For this review, take the finished solid that the model builds, in its own axes (mm). Face numbers are marked on the shaded views. A direction names the side the tool comes from. Give positions to 0.01 mm unless a question says otherwise; leave off trailing zeros. Loops run counter-clockwise (first coordinate to the right, second up) from the corner with the lowest first, then second, coordinate; pieces in that order, holes last. Notation, with made-up numbers: (29, -21.5) - (63, -21.5) arc R22 cw to (63, -10.5) - close; hole circle Ø4 at (83.25, -19). An arc over 180 degrees is marked (long way). Put each result on its own line as item: value.
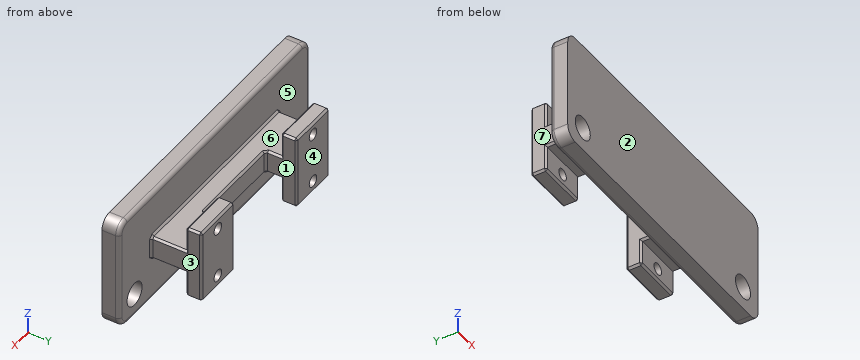
from build123d import *

# Parameters (mm, degrees)
SKETCH1_R                = 3
BOSS_EXTRUDE1_DEPTH      = 4.5
BOSS_EXTRUDE2_DEPTH      = 25.5
BOSS_EXTRUDE2_DEPTH_BACK = 25.5
CUT_EXTRUDE1_DEPTH       = 9.5
CUT_EXTRUDE1_DEPTH_BACK  = 9.5
SKETCH3_W                = 25
SKETCH3_H                = 16
CUT_EXTRUDE2_REACH       = 46.278
SKETCH4_R                = 1.5
FILLET1_R                = 1
CHAMFER1_SIZE            = 0.5


with BuildPart() as part:
    # Sketch1 → Boss-Extrude1 (new body)
    with BuildSketch(Plane(origin=(0, 0, 0), x_dir=(1, 0, 0), z_dir=(0, 1, 0))):
        with BuildLine():
            Line((-35, -14.5), (35, -14.5))
            ThreePointArc((35, -14.5), (37.121320344, -13.621320344), (38, -11.5))
            Line((38, -11.5), (38, 11.5))
            ThreePointArc((38, 11.5), (37.121320344, 13.621320344), (35, 14.5))
            Line((35, 14.5), (-35, 14.5))
            ThreePointArc((-35, 14.5), (-37.121320344, 13.621320344), (-38, 11.5))
            Line((-38, 11.5), (-38, -11.5))
            ThreePointArc((-38, -11.5), (-37.121320344, -13.621320344), (-35, -14.5))
        make_face()
        with Locations(Location((-32, 8.5, 0), (0, 0, 270))):
            Circle(SKETCH1_R, mode=Mode.SUBTRACT)
        with Locations(Location((32, 8.5, 0), (0, 0, 270))):
            Circle(SKETCH1_R, mode=Mode.SUBTRACT)
    extrude(amount=BOSS_EXTRUDE1_DEPTH)

    # Sketch2 → Boss-Extrude2 (add, two sides: drawn at the far end of the back side and taken through both)
    with BuildSketch(Plane(origin=(0, 0, 0), x_dir=(0, 0, -1), z_dir=(1, 0, 0)).offset(-BOSS_EXTRUDE2_DEPTH_BACK)):
        Polygon((-3, 4.5), (-3, 13.5), (-9.5, 13.5), (-9.5, 17.5), (9.5, 17.5), (9.5, 13.5), (3, 13.5), (3, 4.5), align=None)
    extrude(amount=BOSS_EXTRUDE2_DEPTH + BOSS_EXTRUDE2_DEPTH_BACK)

    # Sketch3 → Cut-Extrude1 (cut, two sides: drawn at the far end of the back side and taken through both)
    with BuildSketch(Plane.XY.offset(-CUT_EXTRUDE1_DEPTH_BACK)):
        with Locations((0, 17.5)):
            Rectangle(SKETCH3_W, SKETCH3_H)
    extrude(amount=CUT_EXTRUDE1_DEPTH + CUT_EXTRUDE1_DEPTH_BACK, mode=Mode.SUBTRACT)

    # Sketch4 → Cut-Extrude2 (cut, up to next)
    with BuildSketch(Plane(origin=(0, 17.5, 0), x_dir=(1, 0, 0), z_dir=(0, 1, 0)), mode=Mode.PRIVATE) as cut_extrude2_sk1:
        with Locations(Location((-19, 6.5, 0), (0, 0, 270))):
            Circle(SKETCH4_R)
    cut_extrude2_tool1 = extrude(cut_extrude2_sk1.sketch, amount=-CUT_EXTRUDE2_REACH, mode=Mode.PRIVATE) & part.part
    # Sketch4 → Cut-Extrude2 (cut, up to next)
    with BuildSketch(Plane(origin=(0, 17.5, 0), x_dir=(1, 0, 0), z_dir=(0, 1, 0)), mode=Mode.PRIVATE) as cut_extrude2_sk2:
        with Locations(Location((-19, -6.5, 0), (0, 0, 270))):
            Circle(SKETCH4_R)
    cut_extrude2_tool2 = extrude(cut_extrude2_sk2.sketch, amount=-CUT_EXTRUDE2_REACH, mode=Mode.PRIVATE) & part.part
    # Sketch4 → Cut-Extrude2 (cut, up to next)
    with BuildSketch(Plane(origin=(0, 17.5, 0), x_dir=(1, 0, 0), z_dir=(0, 1, 0)), mode=Mode.PRIVATE) as cut_extrude2_sk3:
        with Locations(Location((19, -6.5, 0), (0, 0, 270))):
            Circle(SKETCH4_R)
    cut_extrude2_tool3 = extrude(cut_extrude2_sk3.sketch, amount=-CUT_EXTRUDE2_REACH, mode=Mode.PRIVATE) & part.part
    # Sketch4 → Cut-Extrude2 (cut, up to next)
    with BuildSketch(Plane(origin=(0, 17.5, 0), x_dir=(1, 0, 0), z_dir=(0, 1, 0)), mode=Mode.PRIVATE) as cut_extrude2_sk4:
        with Locations(Location((19, 6.5, 0), (0, 0, 270))):
            Circle(SKETCH4_R)
    cut_extrude2_tool4 = extrude(cut_extrude2_sk4.sketch, amount=-CUT_EXTRUDE2_REACH, mode=Mode.PRIVATE) & part.part
    add(cut_extrude2_tool1.solids().sort_by_distance((-19, 17.5, -6.5))[0], mode=Mode.SUBTRACT)
    add(cut_extrude2_tool2.solids().sort_by_distance((-19, 17.5, 6.5))[0], mode=Mode.SUBTRACT)
    add(cut_extrude2_tool3.solids().sort_by_distance((19, 17.5, 6.5))[0], mode=Mode.SUBTRACT)
    add(cut_extrude2_tool4.solids().sort_by_distance((19, 17.5, -6.5))[0], mode=Mode.SUBTRACT)

    # Fillet1
    fillet1_edges = [part.edges().sort_by_distance(p)[0] for p in [
        (37.121320344, 4.5, 13.621320344),
        (38, 4.5, 0),
        (37.121320344, 4.5, -13.621320344),
        (0, 4.5, -14.5),
        (-37.121320344, 4.5, -13.621320344),
        (-38, 4.5, 0),
        (-37.121320344, 4.5, 13.621320344),
        (0, 4.5, 14.5),
    ]]
    fillet(fillet1_edges, radius=FILLET1_R)

    # Chamfer1
    chamfer1_edges = [part.edges().sort_by_distance(p)[0] for p in [
        (25.5, 9, 3),
        (25.5, 13.5, 6.25),
        (19, 13.5, 9.5),
        (25.5, 15.5, 9.5),
        (19, 17.5, 9.5),
        (25.5, 17.5, 0),
        (19, 17.5, -9.5),
        (25.5, 15.5, -9.5),
        (19, 13.5, -9.5),
        (25.5, 13.5, -6.25),
        (25.5, 9, -3),
        (0, 4.5, -3),
        (25.5, 4.5, 0),
        (0, 4.5, 3),
        (-25.5, 4.5, 0),
        (-25.5, 9, 3),
        (-25.5, 13.5, 6.25),
        (-25.5, 15.5, 9.5),
        (-25.5, 17.5, 0),
        (-25.5, 15.5, -9.5),
        (-25.5, 13.5, -6.25),
        (-25.5, 9, -3),
        (-12.5, 11.5, -3),
        (0, 9.5, -3),
        (12.5, 11.5, -3),
        (-19, 13.5, -9.5),
        (-19, 17.5, -9.5),
        (-19, 17.5, 9.5),
        (-19, 13.5, 9.5),
        (-12.5, 15.5, 9.5),
        (12.5, 15.5, 9.5),
        (12.5, 13.5, 6.25),
        (12.5, 11.5, 3),
        (12.5, 13.5, -6.25),
        (12.5, 15.5, -9.5),
        (12.5, 17.5, 0),
        (12.5, 9.5, 0),
        (0, 9.5, 3),
        (-12.5, 9.5, 0),
        (-12.5, 11.5, 3),
        (-12.5, 13.5, 6.25),
        (-12.5, 17.5, 0),
        (-12.5, 15.5, -9.5),
        (-12.5, 13.5, -6.25),
    ]]
    chamfer(chamfer1_edges, length=CHAMFER1_SIZE)


solid = part.part
1) Take a section at D-D on x = 32. State the section outline as (y, z) points, and give its area (3 significant figures).
Geometry check:
outline: (0, -14.5) - (3.5, -14.5) arc R1 ccw to (4.5, -13.5) - (4.5, -11.5) - (0, -11.5) - close; (0, -5.5) - (4.5, -5.5) - (4.5, 13.5) arc R1 ccw to (3.5, 14.5) - (0, 14.5) - close
area: 103 mm²
2) Take a section at B-B on z = 6.5. State how many separate pieces and enclosed holes the cut face has, and give its area (3 significant figures).
Geometry check:
separate pieces: 5
enclosed holes: 0
area: 421 mm²
3) Draft analysis for pull direction Y (two halves, no side actions). For the marked faces 4, 5, 6 and 7, state which applies: pulls with the +Y half, pulls with the -Y half, needs draft (parallel to the pull), parting line crosses it, or undercut.
Geometry check:
face 4: pulls with the +Y half
face 5: undercut
face 6: undercut
face 7: needs draft
4) Wall thickness on line 1 (X direction, y = 14.5, z = -6.5); line 2 (X direction, y = 1.8, z = -8.5); line 3 (Y direction, x = 11.5, z = -7.75): over which ranges is each line inside the solid? List them lowest first.
Geometry check:
line 1: x = -25.5 to -20.5, -17.5 to -12.5, 12.5 to 17.5, 20.5 to 25.5
line 2: x = -38 to -35, -29 to 29, 35 to 38
line 3: y = 0 to 4.5
5) For the marked faces 1, 2 and 3, list the 3-axis set-ups (+Z, -Z, +X, -X, +Y, -Y) from which the entire face can be reached by the end or side of a thin tool; tool diameter is ignored.
Geometry check:
face 1: +Z, -Z, +Y
face 2: +Z, -Z, +X, -X, -Y
face 3: +Z, -Z, +X, +Y
6) Take a section at C-C on y = 11. State the section outline as (x, z) points.
Geometry check:
outline: (-25.5, -2.5) - (-25, -3) - (-13, -3) - (-12.5, -2.5) - (-12.5, 2.5) - (-13, 3) - (-25, 3) - (-25.5, 2.5) - close; (12.5, -2.5) - (13, -3) - (25, -3) - (25.5, -2.5) - (25.5, 2.5) - (25, 3) - (13, 3) - (12.5, 2.5) - close
7) Insertion check: pin 1 Ø2 at (x, y) = (-18.5, 7) entering from +Z; pin 2 Ø7.5 at (y, z) = (12.5, -1) entering from +X; pin 3 Ø1.8 at (x, z) = (19, 6.5) entering from +Y; pin 4 Ø1 at (y, z) = (6.5, 5) entering from -X. Each pin has a flat end and moves straight along its axis. Give the tip position at first contact, or say it passes through.
Geometry check:
pin 1: stops at z = 3
pin 2: stops at x = 25.5
pin 3: stops at y = 4.5
pin 4: passes through
8) Take a section at A-A on y = 14.75. State the section outline as (x, z) points, and give its area (3 significant figures).
Geometry check:
outline: (-25.5, -9) - (-25, -9.5) - (-13, -9.5) - (-12.5, -9) - (-12.5, 9) - (-13, 9.5) - (-25, 9.5) - (-25.5, 9) - close; (12.5, -9) - (13, -9.5) - (25, -9.5) - (25.5, -9) - (25.5, 9) - (25, 9.5) - (13, 9.5) - (12.5, 9) - close; hole circle Ø3 at (-19, -6.5); hole circle Ø3 at (-19, 6.5); hole circle Ø3 at (19, -6.5); hole circle Ø3 at (19, 6.5)
area: 465 mm²
